For this review, take the finished solid that the model builds, in its own axes (mm). A direction names the side the tool comes from. Give positions to 0.01 mm unless a question says otherwise; leave off trailing zeros. Order: outer loops, then holes, each group sorted by start corner. A loop starts at its lowest first (then second) coordinate and runs counter-clockwise, first axis right, second up.
Item 1: Consider section D-D (y = 496). Give the boundary of the cut face in (x, z).
Item 2: Consider section A-A (y = 174). Give the boundary of the cut face in (x, z), plus the area to 3 significant figures.
Item 3: Machinability: for faces 4 (the cylindrical face through (-183.742, 284.964, 4.93)), 5 (the flat face through (-8, 304, 0)), which of the approach directions +Z, -Z, +X, -X, +Y, -Y give a long, thin tool a straight path to every point of the face, cutting with its end or side? Answer none if there is none.
Item 4: Consider section C-C (x = 184). Give the boundary of the cut face in (y, z), plus the area to 3 significant figures.
Item 5: For P1, Ø3, axis at y = 244, z = 7.5, coming from the +X side; P2, Ø5, axis at x = -67, z = 5, coming from the -Y side; P3, Ø3, axis at y = 187, z = 3.5, coming from the +X side, all flat-tipped, find the tip position at first contact; note any pin that passes through.
Item 6: The part is to be moulded in two halves that separate along X. For faces 1 (the flat face through (-8, 304, 10)), 2 (the cylindrical face through (-13.194, 599.855, 4.93)), 3 (the cylindrical face through (422.964, 135.742, 4.93)), say which applies: released by +X, released by -X, zero draft, split by the parting line, or undercut.
Item 7: For probe 1 along X at (y, z) = (142.5, 4.25); probe 2 along Z at (x, y) = (0, 595); probe 3 along X at (y, z) = (96.5, 1.75), list the stretches that pass through material, from the lowest coordinate up.
Item 8: Consider section B-B (z = 1.75). Give the boundary of the cut face in (x, y), plus the area to 3 significant figures.
Autodesk Inventor part; units mm, degrees
ref_plane "Work Plane1" through (-600, 600, 0) normal (0, -1, 0) x (1, 0, 0)
ref_plane "YZ Plane" through (0, 0, 0) normal (1, 0, 0) x (0, 1, 0)
ref_plane "XZ Plane" through (0, 0, 0) normal (0, 1, 0) x (-1, 0, 0)
sketch "Sketch1" plane through (0, 0, 0) normal (0, 0, 1) x (1, 0, 0)
  arc A0 (600, 0) -> (-600, 0) centre (0, 0) ccw
  line L0 (-600, 0) -> (600, 0)
  point P0 (0, 0)
  dimension "d0" = 1200
extrude "Extrusion1" add sketch "Sketch1" along normal blind 10
sketch "Sketch2" plane through (0, 0, 10) normal (0, 0, 1) x (1, 0, 0)
  line L0 (-600, 0) -> (600, 0)
  line L1 (438, 0) -> (-198, 0)
  line L2 (-198, 0) -> (-198, 300)
  line L3 (-198, 300) -> (438, 300)
  line L4 (438, 300) -> (438, 0)
  point P0 (0, 0)
  dimension "d3" = 300
  dimension "d4" = 636
  dimension "d5" = 198
extrude "Extrusion2" cut sketch "Sketch2" against normal through all
sketch "Sketch3" plane through (0, 0, 10) normal (0, 0, 1) x (1, 0, 0)
  line L0 (-198, 300) -> (438, 300)
  line L1 (438, 300) -> (52, 300)
  line L2 (52, 300) -> (52, 150)
  line L3 (52, 150) -> (438, 150)
  line L4 (438, 150) -> (438, 300)
  line L5 (-198, 0) -> (-198, 300)
  point P0 (0, 0)
  dimension "d9" = 150
  dimension "d10" = 250
extrude "Extrusion3" add sketch "Sketch3" against normal up to surface (10 mm away)
fillet "Fillet2" radius 50 3 edges at (-198, 300, 5) (52, 300, 5) (438, 150, 5)
ref_plane "Work Plane1" through (-600, 600, 0) normal (0, -1, 0) x (1, 0, 0)
sketch "Sketch4" plane through (-600, 600, 0) normal (0, -1, 0) x (1, 0, 0)
  line L0 (1200, 10) -> (0, 10)
  line L1 (600, 12) -> (600, -2)
  point P0 (600, 0)
  point P1 (600, 5)
  dimension "d15" = 5
hole "Hole1" at (0, 600, 5) direction (0, -1, 0) diameter 3.242 depth 11.8 tip angle 118
pattern_circular "Circular Pattern1" count 14 over 360 about axis through (0, 0, -10) along (0, 0, 1) of "Hole1"
properties part number "Top_Guard 2" material "PMMA Plastic"
Resolved:
1. outline: (-337.62, 0) - (337.62, 0) - (337.62, 10) - (-337.62, 10) - close
2. outline: (-574.22, 0) - (-198, 0) - (-198, 10) - (-574.22, 10) - close; (52, 0) - (574.22, 0) - (574.22, 10) - (52, 10) - close
2. area: 8,980 mm2
3. face 4: +Z, -Z, -Y
3. face 5: -Z, +X, -X, +Y, -Y
4. outline: (150, 0) - (571.09, 0) - (571.09, 10) - (150, 10) - close
4. area: 4,210 mm2
5. P1: stops at x = 548.81
5. P2: stops at y = 300
5. P3: stops at x = 570.6
6. face 1: zero draft
6. face 2: split by the parting line
6. face 3: undercut
7. probe 1: x = -582.83 to -198, 414.34 to 582.83
7. probe 2: z = 0 to 3.38, 6.62 to 10
7. probe 3: x = -592.19 to -198, 438 to 592.19
8. outline: (-600, 0) - (-198, 0) - (-198, 250) arc R50 cw to (-148, 300) - (2, 300) arc R50 cw to (52, 250) - (52, 150) - (388, 150) arc R50 cw to (438, 100) - (438, 0) - (600, 0) arc R600 ccw to start
8. area: 434,000 mm2
